The listing builds one solid part. Answer for the finished solid, in the listing's coordinates (mm). A direction names the side the tool comes from. Round coordinates to 2 decimals unless told otherwise and drop trailing zeros. Write each loop counter-clockwise with the first axis right and the second up, starting at its lowest first coordinate (ties: lowest second). Pieces come first, ordered by that corner, then holes. Notation, with made-up numbers: (-33, 41) -> (13, 41) arc R17 cw to (13, 56) -> close; hole circle Ø7 at (27.5, 74.5). An arc over 180 degrees is marked (long way). Write each question's results on one line, items separated by ' | '. Start each with the question number.
```python
from build123d import *

# Parameters (mm, degrees)
BOSS_EXTRUDE1_DEPTH = 1.5
BOSS_EXTRUDE2_START = 6.55
BOSS_EXTRUDE2_DEPTH = 6.55
SKETCH4_W           = 11.085213563
SKETCH4_H           = 3
SKETCH4_W_2         = 13.3
BOSS_EXTRUDE4_DEPTH = 1
CUT_EXTRUDE1_DEPTH  = 2.2
FILLET1_R           = 1


with BuildPart() as part:
    # Sketch2 → Boss-Extrude1 (new body)
    with BuildSketch(Plane.XY):
        with BuildLine():
            Line((-15.064293146, -76.617402573), (-4.394293146, -76.617402573))
            Line((-4.394293146, -76.617402573), (41.275706854, -76.617402573))
            ThreePointArc((41.275706854, -76.617402573), (43.397027197, -75.738722916), (44.275706854, -73.617402573))
            Line((44.275706854, -73.617402573), (44.275706854, -4.577402573))
            ThreePointArc((44.275706854, -4.577402573), (43.689920416, -3.16318901), (42.275706854, -2.577402573))
            Line((42.275706854, -2.577402573), (40.220988228, -2.577402573))
            ThreePointArc((40.220988228, -2.577402573), (39.455621363, -2.425161638), (38.806774666, -1.991616135))
            Line((38.806774666, -1.991616135), (37.438347541, -0.62318901))
            ThreePointArc((37.438347541, -0.62318901), (36.789500843, -0.189643508), (36.024133979, -0.037402573))
            Line((36.024133979, -0.037402573), (1.601279729, -0.037402573))
            ThreePointArc((1.601279729, -0.037402573), (0.835912864, -0.189643508), (0.187066167, -0.62318901))
            Line((0.187066167, -0.62318901), (-1.181360958, -1.991616135))
            ThreePointArc((-1.181360958, -1.991616135), (-1.830207656, -2.425161638), (-2.59557452, -2.577402573))
            Line((-2.59557452, -2.577402573), (-15.064293146, -2.577402573))
            ThreePointArc((-15.064293146, -2.577402573), (-16.478506709, -3.16318901), (-17.064293146, -4.577402573))
            Line((-17.064293146, -4.577402573), (-17.064293146, -74.617402573))
            ThreePointArc((-17.064293146, -74.617402573), (-16.478506709, -76.031616135), (-15.064293146, -76.617402573))
        make_face()
        with BuildLine():
            Line((5.015493291, -59.617402573), (24.015493291, -59.617402573))
            ThreePointArc((24.015493291, -59.617402573), (26.136813635, -58.738722916), (27.015493291, -56.617402573))
            Line((27.015493291, -56.617402573), (27.015493291, -6.037402573))
            ThreePointArc((27.015493291, -6.037402573), (26.136813635, -3.916082229), (24.015493291, -3.037402573))
            Line((24.015493291, -3.037402573), (12.735677005, -3.037402573))
            ThreePointArc((12.735677005, -3.037402573), (10.614356661, -3.916082229), (9.735677005, -6.037402573))
            Line((9.735677005, -6.037402573), (9.735677005, -11.358022899))
            ThreePointArc((9.735677005, -11.358022899), (8.271210911, -14.893556805), (4.735677005, -16.358022899))
            Line((4.735677005, -16.358022899), (4.015493291, -16.358022899))
            ThreePointArc((4.015493291, -16.358022899), (2.601279729, -16.943809336), (2.015493291, -18.358022899))
            Line((2.015493291, -18.358022899), (2.015493291, -56.617402573))
            ThreePointArc((2.015493291, -56.617402573), (2.894172948, -58.738722916), (5.015493291, -59.617402573))
        make_face(mode=Mode.SUBTRACT)
    extrude(amount=BOSS_EXTRUDE1_DEPTH)

    # Sketch3 → Boss-Extrude2 (add)
    with BuildSketch(Plane(origin=(0, 0, 0), x_dir=(-1, 0, 0), z_dir=(0, 0, -1)).offset(BOSS_EXTRUDE2_START)):
        with BuildLine():
            Line((4.394293146, -75.117402573), (4.394293146, -73.617402573))
            Line((4.394293146, -73.617402573), (14.064293146, -73.617402573))
            Line((14.064293146, -73.617402573), (14.064293146, -5.577402573))
            Line((14.064293146, -5.577402573), (0.524506709, -5.577402573))
            Line((0.524506709, -5.577402573), (-2.015493291, -3.037402573))
            Line((-2.015493291, -3.037402573), (-35.609920416, -3.037402573))
            Line((-35.609920416, -3.037402573), (-38.149920416, -5.577402573))
            Line((-38.149920416, -5.577402573), (-41.275706854, -5.577402573))
            Line((-41.275706854, -5.577402573), (-41.275706854, -73.617402573))
            Line((-41.275706854, -73.617402573), (-38.100706854, -73.617402573))
            Line((-38.100706854, -73.617402573), (-38.100706854, -75.117402573))
            Line((-38.100706854, -75.117402573), (-38.100706854, -76.617402573))
            Line((-38.100706854, -76.617402573), (-41.275706854, -76.617402573))
            ThreePointArc((-41.275706854, -76.617402573), (-43.397027197, -75.738722916), (-44.275706854, -73.617402573))
            Line((-44.275706854, -73.617402573), (-44.275706854, -4.577402573))
            ThreePointArc((-44.275706854, -4.577402573), (-43.689920416, -3.16318901), (-42.275706854, -2.577402573))
            Line((-42.275706854, -2.577402573), (-40.220988228, -2.577402573))
            ThreePointArc((-40.220988228, -2.577402573), (-39.455621363, -2.425161638), (-38.806774666, -1.991616135))
            Line((-38.806774666, -1.991616135), (-37.438347541, -0.62318901))
            ThreePointArc((-37.438347541, -0.62318901), (-36.789500843, -0.189643508), (-36.024133979, -0.037402573))
            Line((-36.024133979, -0.037402573), (-1.601279729, -0.037402573))
            ThreePointArc((-1.601279729, -0.037402573), (-0.835912864, -0.189643508), (-0.187066167, -0.62318901))
            Line((-0.187066167, -0.62318901), (1.181360958, -1.991616135))
            ThreePointArc((1.181360958, -1.991616135), (1.830207656, -2.425161638), (2.59557452, -2.577402573))
            Line((2.59557452, -2.577402573), (15.064293146, -2.577402573))
            ThreePointArc((15.064293146, -2.577402573), (16.478506709, -3.16318901), (17.064293146, -4.577402573))
            Line((17.064293146, -4.577402573), (17.064293146, -74.617402573))
            ThreePointArc((17.064293146, -74.617402573), (16.478506709, -76.031616135), (15.064293146, -76.617402573))
            Line((15.064293146, -76.617402573), (4.394293146, -76.617402573))
            Line((4.394293146, -76.617402573), (4.394293146, -75.117402573))
        make_face()
        Polygon((-8.905706854, -76.617402573), (-8.905706854, -73.617402573), (-27.015493291, -73.617402573), (-27.100706854, -76.617402573), align=None)
    extrude(amount=-BOSS_EXTRUDE2_DEPTH)

    # Sketch4 → Boss-Extrude4 (add)
    with BuildSketch(Plane(origin=(0, 0, 0), x_dir=(-1, 0, 0), z_dir=(0, 0, -1))):
        with Locations((-32.558100073, -75.117402573)):
            Rectangle(SKETCH4_W, SKETCH4_H)
        with Locations((-2.255706854, -75.117402573)):
            Rectangle(SKETCH4_W_2, SKETCH4_H)
    extrude(amount=BOSS_EXTRUDE4_DEPTH)

    # Sketch6 → Cut-Extrude1 (cut)
    with BuildSketch(Plane(origin=(0, 0, -6.55), x_dir=(-1, 0, 0), z_dir=(0, 0, -1))):
        with BuildLine():
            Line((17.064293146, -4.577402573), (17.064293146, -74.617402573))
            ThreePointArc((17.064293146, -74.617402573), (16.478506709, -76.031616135), (15.064293146, -76.617402573))
            Line((15.064293146, -76.617402573), (4.394293146, -76.617402573))
            Line((4.394293146, -76.617402573), (-8.905706854, -76.617402573))
            Line((-8.905706854, -76.617402573), (-27.100706854, -76.617402573))
            Line((-27.100706854, -76.617402573), (-38.100706854, -76.617402573))
            Line((-38.100706854, -76.617402573), (-41.275706854, -76.617402573))
            ThreePointArc((-41.275706854, -76.617402573), (-43.397027197, -75.738722916), (-44.275706854, -73.617402573))
            Line((-44.275706854, -73.617402573), (-44.275706854, -4.577402573))
            ThreePointArc((-44.275706854, -4.577402573), (-43.689920416, -3.16318901), (-42.275706854, -2.577402573))
            Line((-42.275706854, -2.577402573), (-40.220988228, -2.577402573))
            ThreePointArc((-40.220988228, -2.577402573), (-39.455621363, -2.425161638), (-38.806774666, -1.991616135))
            Line((-38.806774666, -1.991616135), (-37.438347541, -0.62318901))
            ThreePointArc((-37.438347541, -0.62318901), (-36.789500843, -0.189643508), (-36.024133979, -0.037402573))
            Line((-36.024133979, -0.037402573), (-1.601279729, -0.037402573))
            ThreePointArc((-1.601279729, -0.037402573), (-0.835912864, -0.189643508), (-0.187066167, -0.62318901))
            Line((-0.187066167, -0.62318901), (1.181360958, -1.991616135))
            ThreePointArc((1.181360958, -1.991616135), (1.830207656, -2.425161638), (2.59557452, -2.577402573))
            Line((2.59557452, -2.577402573), (15.064293146, -2.577402573))
            ThreePointArc((15.064293146, -2.577402573), (16.478506709, -3.16318901), (17.064293146, -4.577402573))
        make_face()
        with BuildLine():
            Line((-38.100706854, -74.817402573), (-41.275706854, -74.817402573))
            ThreePointArc((-41.275706854, -74.817402573), (-42.124234991, -74.46593071), (-42.475706854, -73.617402573))
            Line((-42.475706854, -73.617402573), (-42.475706854, -4.577402573))
            ThreePointArc((-42.475706854, -4.577402573), (-42.41712821, -4.435981216), (-42.275706854, -4.377402573))
            Line((-42.275706854, -4.377402573), (-40.220988228, -4.377402573))
            ThreePointArc((-40.220988228, -4.377402573), (-38.766791185, -4.088144796), (-37.53398246, -3.264408341))
            Line((-37.53398246, -3.264408341), (-36.165555335, -1.895981216))
            ThreePointArc((-36.165555335, -1.895981216), (-36.100670665, -1.852626666), (-36.024133979, -1.837402573))
            Line((-36.024133979, -1.837402573), (-1.601279729, -1.837402573))
            ThreePointArc((-1.601279729, -1.837402573), (-1.524743043, -1.852626666), (-1.459858373, -1.895981216))
            Line((-1.459858373, -1.895981216), (-0.091431248, -3.264408341))
            ThreePointArc((-0.091431248, -3.264408341), (1.141377477, -4.088144796), (2.59557452, -4.377402573))
            Line((2.59557452, -4.377402573), (15.064293146, -4.377402573))
            ThreePointArc((15.064293146, -4.377402573), (15.205714502, -4.435981216), (15.264293146, -4.577402573))
            Line((15.264293146, -4.577402573), (15.264293146, -74.617402573))
            ThreePointArc((15.264293146, -74.617402573), (15.205714502, -74.758823929), (15.064293146, -74.817402573))
            Line((15.064293146, -74.817402573), (4.394293146, -74.817402573))
            Line((4.394293146, -74.817402573), (-38.100706854, -74.817402573))
        make_face(mode=Mode.SUBTRACT)
    extrude(amount=-CUT_EXTRUDE1_DEPTH, mode=Mode.SUBTRACT)

    # Fillet1
    fillet1_edges = [part.edges().sort_by_distance(p)[0] for p in [
        (2.601279729, -16.943809336, 1.5),
        (2.015493291, -37.487712736, 1.5),
        (2.894172948, -58.738722916, 1.5),
        (14.515493291, -59.617402573, 1.5),
        (26.136813635, -58.738722916, 1.5),
        (27.015493291, -31.327402573, 1.5),
        (26.136813635, -3.916082229, 1.5),
        (18.375585148, -3.037402573, 1.5),
        (10.614356661, -3.916082229, 1.5),
        (9.735677005, -8.697712736, 1.5),
        (8.271210911, -14.893556805, 1.5),
        (4.375585148, -16.358022899, 1.5),
        (-17.064293146, -39.597402573, 1.5),
        (-16.478506709, -3.16318901, 1.5),
        (-8.829933833, -2.577402573, 1.5),
        (-1.830207656, -2.425161638, 1.5),
        (-0.497147396, -1.307402573, 1.5),
        (0.835912864, -0.189643508, 1.5),
        (18.812706854, -0.037402573, 1.5),
        (36.789500843, -0.189643508, 1.5),
        (38.122561103, -1.307402573, 1.5),
        (39.455621363, -2.425161638, 1.5),
        (41.248347541, -2.577402573, 1.5),
        (43.689920416, -3.16318901, 1.5),
        (44.275706854, -39.097402573, 1.5),
        (43.397027197, -75.738722916, 1.5),
        (13.105706854, -76.617402573, 1.5),
        (-16.478506709, -76.031616135, 1.5),
    ]]
    fillet(fillet1_edges, radius=FILLET1_R)


solid = part.part
```
Q1. The part is cut by section B-B, the plane x = 16.5. Write down the section's boundary in (y, z).
Q2. For faces 1 (the flat face through (18, -74.817, -5)), 2 (the flat face through (-9, -4.377, -5)), 3 (the flat face through (41.276, -39, -3)), 4 (the cylindrical face through (2.617, -16.928, 0.246)), 5 (the flat face through (8.906, -75, -3)), determine the directions among +Z, -Z, +X, -X, +Y, -Y from which every point of the face is accessible in a straight line to the end or side of a thin tool.
Q3. Determine the mould class of faces 6 (the cylindrical face through (-0.294, -1.53, 1.215)), 7 (the flat face through (19, -3.037, -3)), 8 (the flat face through (-10, -74.817, -5)), 9 (the flat face through (44.276, -40, -2)) for opening direction Y: pulls with the +Y half, pulls with the -Y half, needs draft (parallel to the pull), parting line crosses it, or undercut.
Q4. Each of these flat-tipped pins is pushed along its axis until it touches: pin 1 (4 mm diameter, centred on x = 13.5, y = -57, fed in from -Z); pin 2 (2.5 mm diameter, centred on x = 3, y = -74.5, fed in from -Z); pin 3 (1.5 mm diameter, centred on x = 4, z = -3.5, fed in from -Y); pin 4 (2.5 mm diameter, centred on x = 41.5, z = -3, fed in from +Y). Where does it stop, or does it pass through?
Q5. The part is cut by section A-A, the plane y = -7. Write down the section's boundary in (x, z).
Q6. Find the intervals of material crossed by line 1 (X direction, y = -17.5, z = -4.5); line 2 (X direction, y = -24.5, z = -3.25); line 3 (Y direction, x = -5, z = -0.5), in increasing order.
Q7. The part is cut by section D-D, the plane y = -54. Write down the section's boundary in (x, z), then the cut area to 3 significant figures.
Answers follow:
1) outline: (-76.62, -4.35) -> (-74.82, -4.35) -> (-74.82, -6.55) -> (-73.62, -6.55) -> (-73.62, 0) -> (-59.62, 0) -> (-59.62, 0.5) arc R1 ccw to (-60.62, 1.5) -> (-75.62, 1.5) arc R1 ccw to (-76.62, 0.5) -> close; (-3.04, -6.55) -> (-1.84, -6.55) -> (-1.84, -4.35) -> (-0.04, -4.35) -> (-0.04, 0.5) arc R1 ccw to (-1.04, 1.5) -> (-2.04, 1.5) arc R1 ccw to (-3.04, 0.5) -> close
2) face 1: -Z, +X, -X, -Y | face 2: -Z, -X, +Y | face 3: -Z | face 4: +Z, -Z | face 5: -Z, -Y
3) face 6: pulls with the +Y half | face 7: undercut | face 8: pulls with the -Y half | face 9: needs draft
4) pin 1: through | pin 2: z = -1 | pin 3: y = -3.04 | pin 4: y = -2.58
5) outline: (-17.06, -4.35) -> (-15.26, -4.35) -> (-15.26, -6.55) -> (-14.06, -6.55) -> (-14.06, 0) -> (9.74, 0) -> (9.74, 0.5) arc R1 ccw to (8.74, 1.5) -> (-16.06, 1.5) arc R1 ccw to (-17.06, 0.5) -> close; (27.02, 0) -> (41.28, 0) -> (41.28, -6.55) -> (42.48, -6.55) -> (42.48, -4.35) -> (44.28, -4.35) -> (44.28, 0.5) arc R1 ccw to (43.28, 1.5) -> (28.02, 1.5) arc R1 ccw to (27.02, 0.5) -> close
6) line 1: -15.26 to -14.06, 41.28 to 42.48 | line 2: -17.06 to -14.06, 41.28 to 44.28 | line 3: -76.62 to -73.62, -5.58 to -2.58
7) outline: (-17.06, -4.35) -> (-15.26, -4.35) -> (-15.26, -6.55) -> (-14.06, -6.55) -> (-14.06, 0) -> (2.02, 0) -> (2.02, 0.5) arc R1 ccw to (1.02, 1.5) -> (-16.06, 1.5) arc R1 ccw to (-17.06, 0.5) -> close; (27.02, 0) -> (41.28, 0) -> (41.28, -6.55) -> (42.48, -6.55) -> (42.48, -4.35) -> (44.28, -4.35) -> (44.28, 0.5) arc R1 ccw to (43.28, 1.5) -> (28.02, 1.5) arc R1 ccw to (27.02, 0.5) -> close | area: 85.0 mm^2
